from build123d import *

# Parameters (mm, degrees)
SKETCH1_W           = 243.84
SKETCH1_H           = 177.8
SKETCH1_W_2         = 233.68
SKETCH1_H_2         = 167.64
BOSS_EXTRUDE7_DEPTH = 12.7
SKETCH6_W           = 233.68
SKETCH6_H           = 167.64
BOSS_EXTRUDE8_DEPTH = 7.62
CUT_EXTRUDE2_DEPTH  = 8
FILLET1_R           = 2.54


with BuildPart() as part:
    # Sketch1 → Boss-Extrude7 (new body)
    with BuildSketch(Plane(origin=(0, 0, 0), x_dir=(1, 0, 0), z_dir=(0, 1, 0))):
        with Locations((121.92, 88.9)):
            Rectangle(SKETCH1_W, SKETCH1_H)
        with Locations((121.92, 88.9)):
            Rectangle(SKETCH1_W_2, SKETCH1_H_2, mode=Mode.SUBTRACT)
    extrude(amount=BOSS_EXTRUDE7_DEPTH)

    # Sketch6 → Boss-Extrude8 (add)
    with BuildSketch(Plane(origin=(0, 12.7, 0), x_dir=(1, 0, 0), z_dir=(0, 1, 0))):
        with Locations((121.92, 88.9)):
            Rectangle(SKETCH6_W, SKETCH6_H)
    extrude(amount=-BOSS_EXTRUDE8_DEPTH)

    # Sketch7 → Cut-Extrude2 (cut)
    with BuildSketch(Plane(origin=(0, 12.7, 0), x_dir=(1, 0, 0), z_dir=(0, 1, 0))):
        Polygon((196.37, 1.27), (178.258137899, 1.27), (178.258137899, 0), (168.098137899, 0), (168.098137899, 1.27), (157.995367116, 1.27), (47.47, 1.27), (47.47, 63.07), (145.57, 63.07), (145.57, 64.34), (183.67, 64.34), (183.67, 63.07), (196.37, 63.07), align=None)
    extrude(amount=-CUT_EXTRUDE2_DEPTH, mode=Mode.SUBTRACT)

    # Fillet1
    fillet1_edges = [part.edges().sort_by_distance(p)[0] for p in [
        (47.47, 8.89, -63.07),
        (47.47, 8.7, -1.27),
        (196.37, 8.89, -63.07),
        (196.37, 8.7, -1.27),
    ]]
    fillet(fillet1_edges, radius=FILLET1_R)


solid = part.part
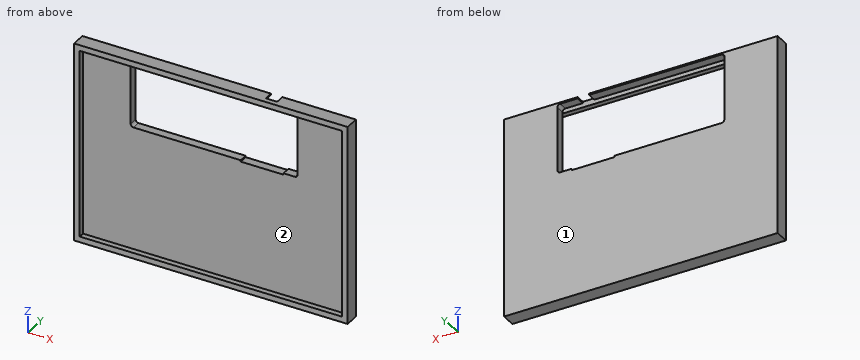
Check sheet for the modelled part. Datum: model origin and axes. Units: mm. Face numbers are marked on the shaded views. Round coordinates to 2 decimals unless told otherwise and drop trailing zeros. Order: outer loops, then holes, each group sorted by start corner. A loop starts at its lowest first (then second) coordinate and runs counter-clockwise, first axis right, second up.
Q1. Cross-section at B-B, the plane z = -43. Enter the section's corners in (x, y).
Filled sheet:
outline: (0, 0) - (5.08, 0) - (5.08, 5.08) - (47.47, 5.08) - (47.47, 12.7) - (0, 12.7) - close; (196.37, 5.08) - (238.76, 5.08) - (238.76, 0) - (243.84, 0) - (243.84, 12.7) - (196.37, 12.7) - close
Q2. Scan lines: L1, parallel to X at y = 4.75, z = -57; L2, parallel to Z at x = 179.5, y = 11.25; L3, parallel to Z at x = 225.5, y = 0.5. Record each from-to range of solid material in increasing order.
Filled sheet:
L1: x = 0 to 5.08, 238.76 to 243.84
L2: z = -177.8 to -64.34, -1.27 to 0
L3: z = -177.8 to -172.72, -5.08 to 0
Q3. Cross-section at D-D, the plane x = 209. Enter the section's corners in (y, z), plus the area to 3 significant figures.
Filled sheet:
outline: (0, -177.8) - (12.7, -177.8) - (12.7, 0) - (0, 0) - (0, -5.08) - (5.08, -5.08) - (5.08, -172.72) - (0, -172.72) - close
area: 1,410 mm2
Q4. Cross-section at A-A, the plane x = 65.5. Enter the section's corners in (y, z), plus the area to 3 significant figures.
Filled sheet:
outline: (0, -177.8) - (12.7, -177.8) - (12.7, -63.07) - (5.08, -63.07) - (5.08, -172.72) - (0, -172.72) - close; (0, -5.08) - (4.7, -5.08) - (4.7, -1.27) - (12.7, -1.27) - (12.7, 0) - (0, 0) - close
area: 934 mm2
Q5. Depth check by flat-ended pin: P1, Ø4, axis at x = 113, z = -3.5, coming from the +Y side. Enter the tip coordinate at first touch or a pass-through.
Filled sheet:
P1: stops at y = 4.7
Q6. Cross-section at C-C, the plane z = -116. Enter the section's corners in (x, y), plus the area to 3 significant figures.
Filled sheet:
outline: (0, 0) - (5.08, 0) - (5.08, 5.08) - (238.76, 5.08) - (238.76, 0) - (243.84, 0) - (243.84, 12.7) - (0, 12.7) - close
area: 1,910 mm2
Q7. Draft check along Z on the marked faces 1 and 2. Enter one of: pulls with the +Z half, pulls with the -Z half, needs draft (parallel to the pull), parting line crosses it, or undercut.
Filled sheet:
face 1: needs draft
face 2: undercut
